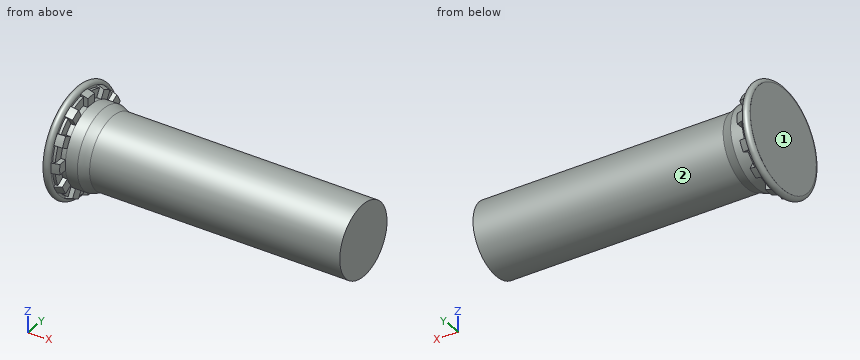
```python
from build123d import *

# Parameters (mm, degrees)
RIBCUT1_DEPTH    = 0.31875
RIBCUT2_DEPTH    = 0.51
RIBCUTSPAT_COUNT = 12
RIBCUTSPAT_ANGLE = 330


with BuildPart() as part:
    # BodySke → BaseBody (revolve)
    with BuildSketch(Plane.XY, mode=Mode.PRIVATE) as basebody_sk:
        with BuildLine():
            Line((0, 0), (0, 3.49246))
            Line((0, 3.49246), (0.00508, 3.49246))
            Line((0.00508, 3.49246), (0.00508, 3.49754))
            ThreePointArc((0.00508, 3.49754), (0.25754, 3.75), (0.51, 3.49754))
            Line((0.51, 3.49754), (0.51, 3.4925))
            Line((0.51, 3.4925), (1.02, 3.343625))
            Line((1.02, 3.343625), (1.02, 2.75))
            Line((1.02, 2.75), (1.863130645, 2.75))
            Line((1.863130645, 2.75), (2.55, 2.5))
            Line((2.55, 2.5), (20, 2.5))
            Line((20, 2.5), (20, 0))
            Line((20, 0), (0, 0))
        make_face()
    revolve(basebody_sk.sketch.rotate(Axis((0, 0, 0), (1, 0, 0)), 90), axis=Axis((0, 0, 0), (1, 0, 0)))

    # RibCut1Ske → RibCut1 (cut)
    with BuildSketch(Plane(origin=(1.02, 0, 0), x_dir=(0, 0, -1), z_dir=(1, 0, 0))):
        with BuildLine():
            Line((0.358947029, 2.726473369), (0.358947029, 3.732781407))
            ThreePointArc((0.358947029, 3.732781407), (0.970571419, 3.622221849), (1.555533458, 3.412157039))
            Line((1.555533458, 3.412157039), (1.052379439, 2.540668714))
            ThreePointArc((1.052379439, 2.540668714), (0.711752374, 2.656296022), (0.358947029, 2.726473369))
        make_face()
    ribcut1 = extrude(amount=-RIBCUT1_DEPTH, mode=Mode.SUBTRACT)

    # RibCut2Ske → RibCut2 (cut)
    with BuildSketch(Plane(origin=(1.02, 0, 0), x_dir=(0, 0, -1), z_dir=(1, 0, 0))):
        with BuildLine():
            Line((0.358947029, 3.324302208), (0.358947029, 3.732781407))
            ThreePointArc((0.358947029, 3.732781407), (0.970571419, 3.622221849), (1.555533458, 3.412157039))
            Line((1.555533458, 3.412157039), (1.351293859, 3.058403676))
            ThreePointArc((1.351293859, 3.058403676), (0.86539383, 3.229693741), (0.358947029, 3.324302208))
        make_face()
    ribcut2 = extrude(amount=-RIBCUT2_DEPTH, mode=Mode.SUBTRACT)

    # RibCutsPat: RibCut1, RibCut2 ×12 about axis
    ribcutspat_axis = Axis((0, 0, 0), (1, 0, 0))
    add([ribcut1.rotate(ribcutspat_axis, i * RIBCUTSPAT_ANGLE / (RIBCUTSPAT_COUNT - 1)) for i in range(1, RIBCUTSPAT_COUNT)], mode=Mode.SUBTRACT)
    add([ribcut2.rotate(ribcutspat_axis, i * RIBCUTSPAT_ANGLE / (RIBCUTSPAT_COUNT - 1)) for i in range(1, RIBCUTSPAT_COUNT)], mode=Mode.SUBTRACT)


solid = part.part
```
Input: part model. Units: mm. Frame: model coordinates. Face numbers are marked on the shaded views. A direction names the side the tool comes from. Give positions to 0.01 mm unless a question says otherwise; leave off trailing zeros. Order: outer loops, then holes, each group sorted by start corner. A loop starts at its lowest first (then second) coordinate and runs counter-clockwise, first axis right, second up.
1. Pin query (flat end, axial travel): pin 1 Ø1.5 at (x, y) = (9, 2.5) entering from -Z; pin 2 Ø0.7 at (y, z) = (3, -1.5) entering from +X; pin 3 Ø3 at (x, y) = (4.5, -0.5) entering from +Z. Return the tip coordinate at first contact, or that it passes through.
Computed:
pin 1: stops at z = -1.79
pin 2: stops at x = 1.02
pin 3: stops at z = 2.5
2. Line query: probe 1 along X at (y, z) = (3.25, 0.5); probe 2 along Y at (x, z) = (9, 0); probe 3 along Y at (x, z) = (10.75, -2). Output: solid intervals per line, ascending.
Computed:
probe 1: x = 0 to 0.7
probe 2: y = -2.5 to 2.5
probe 3: y = -1.5 to 1.5
3. Cut plane C-C (x = 16.75). Return loops of the section in (y, z), and give its area (3 significant figures).
Computed:
outline: circle Ø5 at (0, 0)
area: 19.6 mm2
4. Set-up query: the marked faces 1 and 2. Return all of +Z, -Z, +X, -X, +Y, -Y with unobstructed straight access to the full face (end or side cutting, diameter ignored); none if empty.
Computed:
face 1: +Z, -Z, -X, +Y, -Y
face 2: +X
